CAD build for the part. Positions are in the model's coordinates, mm. A direction names the side the tool comes from. Coordinates: 2 decimals unless noted, no trailing zeros. Write each loop counter-clockwise with the first axis right and the second up, starting at its lowest first coordinate (ties: lowest second). Pieces come first, ordered by that corner, then holes. Notation, with made-up numbers: (41, 18) -> (95, 18) arc R29 cw to (95, 46) -> close; hole circle Ø10 at (40.5, -6.5). An arc over 180 degrees is marked (long way). Answer as CSV lines item,"result". Start each with the question number.
```python
from build123d import *

# Parameters (mm, degrees)
F0_W     = 444.5
F0_H     = 406.4
F0_W_2   = 419.1
F0_H_2   = 381
F1_DEPTH = 63.5
F2_W     = 419.1
F2_H     = 381
F3_DEPTH = 12.7
F4_W     = 419.1
F4_H     = 381
F5_DEPTH = 6.35
F6_DEPTH = 38.1


with BuildPart() as f1:
    # F0 (on Top) → F1 (new body)
    with BuildSketch(Plane.XY):
        Rectangle(F0_W, F0_H)
        Rectangle(F0_W_2, F0_H_2, mode=Mode.SUBTRACT)
    extrude(amount=F1_DEPTH)

    # F2 (on face) → F3 (join)
    with BuildSketch(Plane(origin=(0, 0, 0), x_dir=(1, 0, 0), z_dir=(0, 0, -1))):
        Rectangle(F2_W, F2_H)
    extrude(amount=-F3_DEPTH)

    # F4 (on face) → F5 (cut)
    with BuildSketch(Plane(origin=(0, 0, 0), x_dir=(1, 0, 0), z_dir=(0, 0, -1))):
        Rectangle(F4_W, F4_H)
    extrude(amount=-F5_DEPTH, mode=Mode.SUBTRACT)

    # F6 (add): a face of the model
    f6_faces = [f1.faces().sort_by_distance(p)[0] for p in [
        (216.2271999037, 0, 63.5),
    ]]
    extrude(f6_faces, amount=F6_DEPTH)


solid = f1.part
```
1. Cut at B-B (y = -149). Give the cut face in (x, z), then the cut area to 3 significant figures.
2. Wall check: line 1 (X direction, y = -101.5, z = 24.5); line 2 (Y direction, x = 5.5, z = 97); line 3 (Z direction, x = -116, y = -14.5). Give the ranges that are in metal, low to high.
3. Mould opens along X. For faces 1 (the face through (222.25, -3, 50)), 2 (the face through (-222.25, -3, 50)), 3 (the face through (-3, 190.5, 57)), 4 (the face through (-18, 195, 0)) say: pulls with the +X half, pulls with the -X half, needs draft (parallel to the pull), parting line crosses it, or undercut.
4. Flat gauge pin, fed straight in: P1, Ø12, axis at x = -157.5, y = 112.5, coming from the +Z side. Where does the tip first touch, or does it go through?
5. Cut at C-C (x = -101.5). Give the cut face in (y, z).
6. Cut at A-A (z = 35.5). Give the cut face in (x, y).
7. Tool access for faces 5 (the face through (-3, 203.2, 50)), 6 (the face through (-3, -3, 6.35)), 7 (the face through (209.55, -3, 57)): list every direction of +Z, -Z, +X, -X, +Y, -Y with a clear straight run to the whole face (end or side of a thin tool).
Geometry check:
1,outline,"(-222.25, 0) -> (-209.55, 0) -> (-209.55, 6.35) -> (209.55, 6.35) -> (209.55, 0) -> (222.25, 0) -> (222.25, 101.6) -> (209.55, 101.6) -> (209.55, 12.7) -> (-209.55, 12.7) -> (-209.55, 101.6) -> (-222.25, 101.6) -> close"
1,area,"5,240 mm²"
2,line 1,"-222.25 to -209.55, 209.55 to 222.25"
2,line 2,"-203.2 to -190.5, 190.5 to 203.2"
2,line 3,"6.35 to 12.7"
3,face 1,"pulls with the +X half"
3,face 2,"pulls with the -X half"
3,face 3,"undercut"
3,face 4,"needs draft"
4,P1,"z = 12.7"
5,outline,"(-203.2, 0) -> (-190.5, 0) -> (-190.5, 6.35) -> (190.5, 6.35) -> (190.5, 0) -> (203.2, 0) -> (203.2, 101.6) -> (190.5, 101.6) -> (190.5, 12.7) -> (-190.5, 12.7) -> (-190.5, 101.6) -> (-203.2, 101.6) -> close"
6,outline,"(-222.25, -203.2) -> (222.25, -203.2) -> (222.25, 203.2) -> (-222.25, 203.2) -> close; hole (-209.55, -190.5) -> (209.55, -190.5) -> (209.55, 190.5) -> (-209.55, 190.5) -> close"
7,face 5,"+Z, -Z, +X, -X, +Y"
7,face 6,"-Z"
7,face 7,"+Z"
